Autodesk Inventor part; units mm, degrees
ref_plane "YZ Plane" through (0, 0, 0) normal (1, 0, 0) x (0, 1, 0)
ref_plane "XZ Plane" through (0, 0, 0) normal (0, 1, 0) x (-1, 0, 0)
ref_plane "XY Plane" through (0, 0, 0) normal (0, 0, 1) x (1, 0, 0)
sketch "Эскиз3" plane through (0, 0, 0) normal (0, 0, 1) x (1, 0, 0)
  line L0 (26, 0) -> (48.5118, 0)
  line L1 (48.5118, 0) -> (48.5118, 16.4882)
  line L2 (26, 15) -> (18, 15)
  line L3 (18, 15) -> (18, 27)
  line L4 (18, 27) -> (38, 27)
  line L5 (38, 27) -> (48.5118, 16.4882)
  line L6 (38, 27) -> (52.866, 27) construction
  line L7 (26, 15) -> (26, 0)
  dimension "d18" = 14.866
  dimension "d19" = 45
  dimension "d20" = 20
  dimension "d25" = 8
sketch "Эскиз4" plane through (0, 0, 0) normal (0, 1, 0) x (-1, 0, 0)
  arc A0 (-24.7386, 8) -> (-24.7386, -8) centre (0, 0) ccw
  dimension "d31" = 26
sweep "Сдвиг1" add profiles "Эскиз3" path "Эскиз4"
sketch "Эскиз5" plane through (0, 0, 0) normal (0, -1, 0) x (1, 0, 0)
  arc A0 (36.1565, 11.6923) -> (36.1565, -11.6923) centre (0, 0) ccw
  circle A1 centre (38, 0) radius 1.575
  point P0 (0, 0)
  dimension "d27" = 3.15
extrude "Выдавливание2" cut sketch "Эскиз5" against normal up to surface (27 mm away)
sketch "Эскиз7" plane through (46.1583, 0, 14.9267) normal (-0.3076923, 0, 0.9514859) x (0.9514859, 0, 0.3076923)
  line L0 (-13.9304, 0) -> (-13.9304, 27)
  line L1 (-10.7804, 0) -> (-10.7804, 25.4984)
  line L2 (-13.9304, 0) -> (-10.7804, 0)
  line L3 (-12.3554, 12.4) -> (-12.3554, 0) construction
  line L4 (-22.5118, 0) -> (0, 0)
  line L5 (-15.1554, 8.4) -> (-9.5554, 8.4)
  line L6 (-9.5554, 8.4) -> (-9.5554, 6)
  line L7 (-9.5554, 6) -> (-15.1554, 6)
  line L8 (-15.1554, 6) -> (-15.1554, 8.4)
  line L9 (-9.5554, 6) -> (-15.1554, 8.4) construction
  point P0 (-48.5118, 0)
  point P1 (-12.3554, 7.2)
  dimension "d35" = 5.6
  dimension "d36" = 2.4
  dimension "d37" = 1.575
  dimension "d38" = 6
extrude "Выдавливание3" cut sketch "Эскиз7" against normal blind 14 contours L7 L8 L5 L0 | L0 L5 L1 L7 | L1 L5 L6 L7
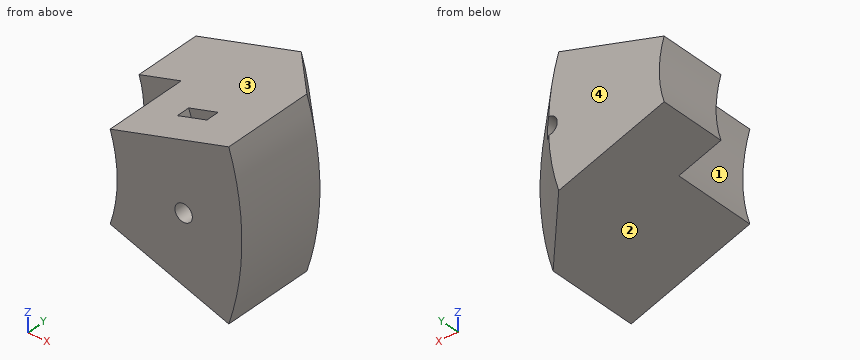
Input: part model. Units: mm. Frame: model coordinates. Face numbers are marked on the shaded views. Coordinates: 2 decimals unless noted, no trailing zeros. Loops run counter-clockwise (first coordinate to the right, second up) from the corner with the lowest first, then second, coordinate; pieces in that order, holes last.
(1) Pull-direction query (Z, two-part tool) for the marked faces 1, 2, 3 and 4; classes: released by +Z, released by -Z, zero draft, split by the parting line, or undercut.
(2) Section B-B on z = 0. Return the cut outline in (x, y) (3 decimals).
(3) Section A-A on y = 5.25. Return the cut outline in (x, z) (3 decimals).
(4) First-contact query: pin 1 Ø4 at (y, z) = (21, -3.5) entering from +X; pin 2 Ø4 at (y, z) = (12.5, 3) entering from -X; pin 3 Ø10 at (x, z) = (20.5, 3) entering from -Y. Flat tips, straight axial feed; report the tip coordinate or a pass-through.
(5) Section C-C on x = 35. Return the cut outline in (y, z), then the cut area to 3 significant figures.
(6) Section D-D on y = 18.25. Return the cut outline in (x, z) (3 decimals), then the cut area to 3 significant figures.
(7) Material intervals for probe 1 along Y at (x, z) = (35.5, -0.5); probe 2 along Z at (x, y) = (38, 1.75) (3 decimals); probe 3 along Z at (x, y) = (38.5, 18.5), sorted ascending.
Data:
1. face 1: undercut
1. face 2: released by -Z
1. face 3: released by +Z
1. face 4: zero draft
2. outline: (18, 15) - (26, 15) - (26, 0) - (36.425, 0) - (36.425, 6) - (35.057, 6) - (35.057, 8.4) - (36.425, 8.4) - (36.425, 27) - (18, 27) - close; (39.575, 0) - (48.512, 0) - (48.512, 16.488) - (39.575, 25.425) - (39.575, 8.4) - (40.943, 8.4) - (40.943, 6) - (39.575, 6) - close
3. outline: (24.739, -8) - (46.158, -14.927) arc R48.512 ccw to (46.158, 14.927) - (24.739, 8) arc R26 cw to start; hole circle Ø3.15 at (38, 0)
4. pin 1: stops at x = 45.87
4. pin 2: stops at x = 25.51
4. pin 3: stops at y = 15
5. outline: (0, -11.32) - (27, -11.32) - (27, 11.32) - (8.4, 11.32) - (8.4, 0.18) - (6, 0.18) - (6, 11.32) - (0, 11.32) - close
5. area: 584 mm2
6. outline: (17.127, -5.538) - (44.482, -14.385) arc R46.75 ccw to (44.482, 14.385) - (17.127, 5.538) arc R18 cw to start; hole circle Ø3.15 at (38, 0)
6. area: 574 mm2
7. probe 1: y = 0 to 6, 8.4 to 27
7. probe 2: z = -12.288 to -1.575, 1.575 to 12.288
7. probe 3: z = -12.45 to -1.49, 1.49 to 12.45
